```python
from build123d import *

# Parameters (mm, degrees)
F0_W     = 54.9000054598
F0_H     = 38.1000023335
F1_DEPTH = 15
F4_D     = 5.5
F5_R     = 3.7947326362
F6_DEPTH = 25


with BuildPart() as f1:
    # F0 (on Front) → F1 (new body)
    with BuildSketch(Plane.XZ):
        with Locations((2.7000010014, -1.9500004128)):
            Rectangle(F0_W, F0_H)
    extrude(amount=F1_DEPTH)

    # F4 (through all)
    with Locations(Plane(origin=(31.8803364434, -8.5423104044, 0), x_dir=(-0.2588190451, -0.9659258263, 0), z_dir=(0.9659258263, -0.2588190451, 0))):
        with Locations((16.5139008313, 3.4433358815)):
            Hole(F4_D / 2)

    # F5 (on Front) → F6 (cut)
    with BuildSketch(Plane.XZ):
        with Locations((-18.1499999017, 5.7000000961)):
            Circle(F5_R)
    extrude(amount=F6_DEPTH, mode=Mode.SUBTRACT)


solid = f1.part
```
The model under review builds one solid part; all positions refer to its coordinate system, in mm. Round coordinates to 2 decimals unless told otherwise and drop trailing zeros. Loops run counter-clockwise (first coordinate to the right, second up) from the corner with the lowest first, then second, coordinate; pieces in that order, holes last. Notation, with made-up numbers: (-8, 42.5) -> (22, 42.5) arc R30 cw to (22, 78.5) -> close; hole circle Ø1 at (13.5, -33.75). An arc over 180 degrees is marked (long way). Answer in a Markdown table with one row per item.
1) Consider section B-B, the plane y = -4.5. Write out the cut boundary in (x, z), plus the area to 3 significant figures.
Taken from the geometry:
| item | result |
|---|---|
| outline | (-24.75, -21) -> (30.15, -21) -> (30.15, 17.1) -> (-24.75, 17.1) -> close; hole circle Ø7.59 at (-18.15, 5.7) |
| area | 2,050 mm² |
2) For pin 1 Ø7 at (x, z) = (-18.15, 5.7) entering from +Y (3 decimals), flat-tipped, find the tip position at first contact; note if it passes through.
Taken from the geometry:
| item | result |
|---|---|
| pin 1 | passes through |
3) Wall thickness on line 1 along Z through (x, y) = (-18.15, -10.5); line 2 along Z through (x, y) = (-18.15, -6); line 3 along Z through (x, y) = (-18.15, -11.25): over which ranges is each line inside the solid? List them lowest first.
Taken from the geometry:
| item | result |
|---|---|
| line 1 | z = -21 to -5.63, -1.26 to 1.91, 9.49 to 17.1 |
| line 2 | z = -21 to 1.91, 9.49 to 17.1 |
| line 3 | z = -21 to -6.02, -0.86 to 1.91, 9.49 to 17.1 |
4) Draft analysis for pull direction Z (two halves, no side actions). For faces 1 (the flat face through (-24.75, -7, -2)), 2 (the cylindrical face through (-19, -7, 2)), 3 (the flat face through (2, -7, 17.1)), 4 (the cylindrical face through (-14.26, -10.56, -4.27)), state which applies: pulls with the +Z half, pulls with the -Z half, needs draft (parallel to the pull), parting line crosses it, or undercut.
Taken from the geometry:
| item | result |
|---|---|
| face 1 | needs draft |
| face 2 | undercut |
| face 3 | pulls with the +Z half |
| face 4 | undercut |
5) Consider section A-A, the plane z = 5.7. Write out the cut boundary in (x, y), plus the area to 3 significant figures.
Taken from the geometry:
| item | result |
|---|---|
| outline | (-24.75, -15) -> (-21.94, -15) -> (-21.94, 0) -> (-24.75, 0) -> close; (-14.36, -15) -> (30.15, -15) -> (30.15, 0) -> (-14.36, 0) -> close |
| area | 710 mm² |
